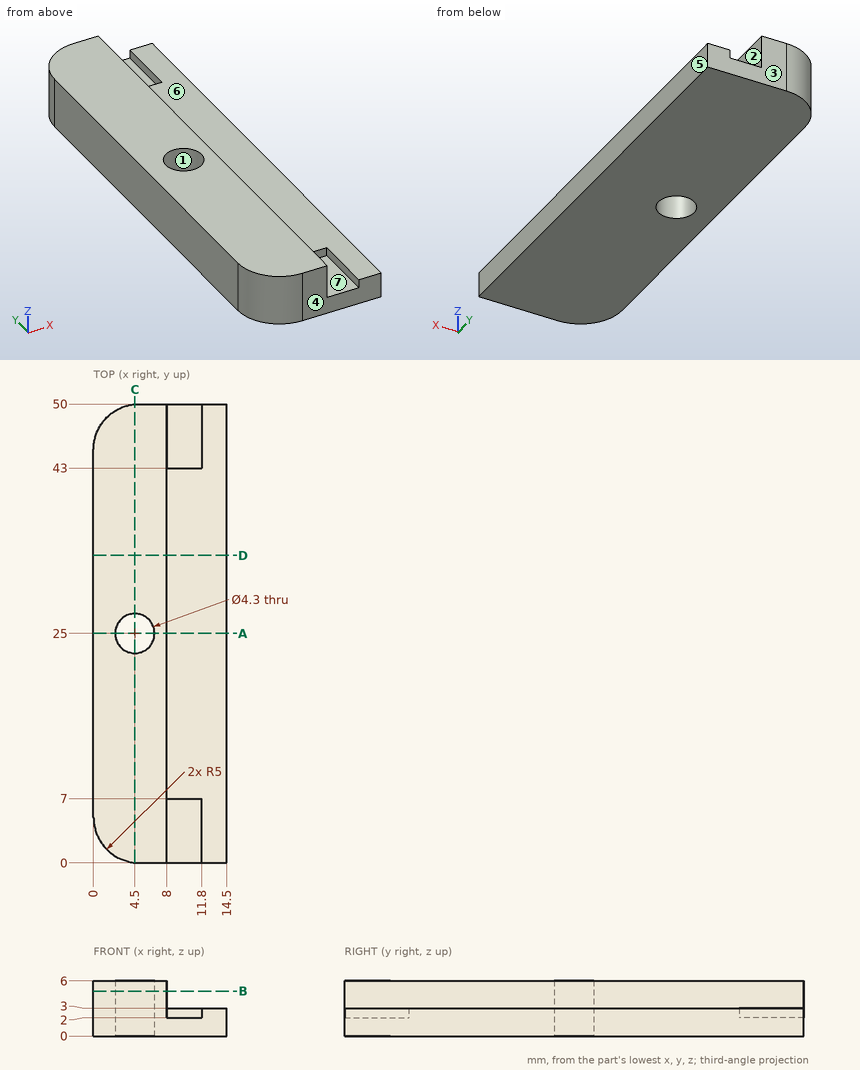
Source: three-view drawing plus pictorial views. Frame: mm from the lowest corner of the part. A direction names the side the tool comes from. Coordinates: 2 decimals unless noted, no trailing zeros. Order: outer loops, then holes, each group sorted by start corner. A loop starts at its lowest first (then second) coordinate and runs counter-clockwise, first axis right, second up. Notation, with made-up numbers: M -6.75,73 L 44.25,73 A21 ccw 44.25,101 Z; hole C 20.5,21.5 d6. An arc over 180 degrees is marked long. Write each question's results on one line, items separated by ' | '. Start each with the question number.
1. Draft query along Y for the marked faces 1, 2, 3 and 4. Return one class per face: +Y half, -Y half, draft (parallel to the pull), parting line (faces both ways), or undercut.
2. Pin query (flat end, axial travel): pin 1 (3 mm diameter, centred on y = 17, z = 5, fed in from +X); pin 2 (0.5 mm diameter, centred on y = 3, z = 2.5, fed in from -X); pin 3 (3 mm diameter, centred on x = 10.5, y = 20, fed in from +Z). Return the tip coordinate at first contact, or that it passes through.
3. Material intervals for L1, parallel to X at y = 28, z = 5.65; L2, parallel to Z at x = 13, y = 23; L3, parallel to Y at x = 5.25, z = 3.8, sorted ascending.
4. Reachability of the marked faces 5, 6 and 7 from +Z, -Z, +X, -X, +Y, -Y: full face, straight path, thin tool, end or side. Return the list, or none.
5. Section D-D, the plane y = 33.5. Return the cut outline in (x, z).
6. Section C-C, the plane x = 4.5. Return the cut outline in (y, z).
7. Section B-B, the plane z = 4.9. Return the cut outline in (x, y), then the cut area to 3 significant figures.
8. Section A-A, the plane y = 25. Return the cut outline in (x, z).
Solution:
1) face 1: undercut | face 2: draft | face 3: +Y half | face 4: -Y half
2) pin 1: x = 8 | pin 2: x = 0.32 | pin 3: z = 3
3) L1: 0 to 8 | L2: 0 to 3 | L3: 0 to 22.99, 27.01 to 50
4) face 5: +Z, -Z, +X, +Y, -Y | face 6: +Z, +X, +Y, -Y | face 7: +Z, -Y
5) outline: M 0,0 L 14.5,0 L 14.5,3 L 8,3 L 8,6 L 0,6 Z
6) outline: M 0.03,0 L 22.85,0 L 22.85,6 L 0.03,6 Z; M 27.15,0 L 49.97,0 L 49.97,6 L 27.15,6 Z
7) outline: M 0,5 A5 ccw 5,0 L 8,0 L 8,50 L 5,50 A5 ccw 0,45 Z; hole C 4.5,25 d4.3 | area: 375 mm²
8) outline: M 0,0 L 2.35,0 L 2.35,6 L 0,6 Z; M 6.65,0 L 14.5,0 L 14.5,3 L 8,3 L 8,6 L 6.65,6 Z
